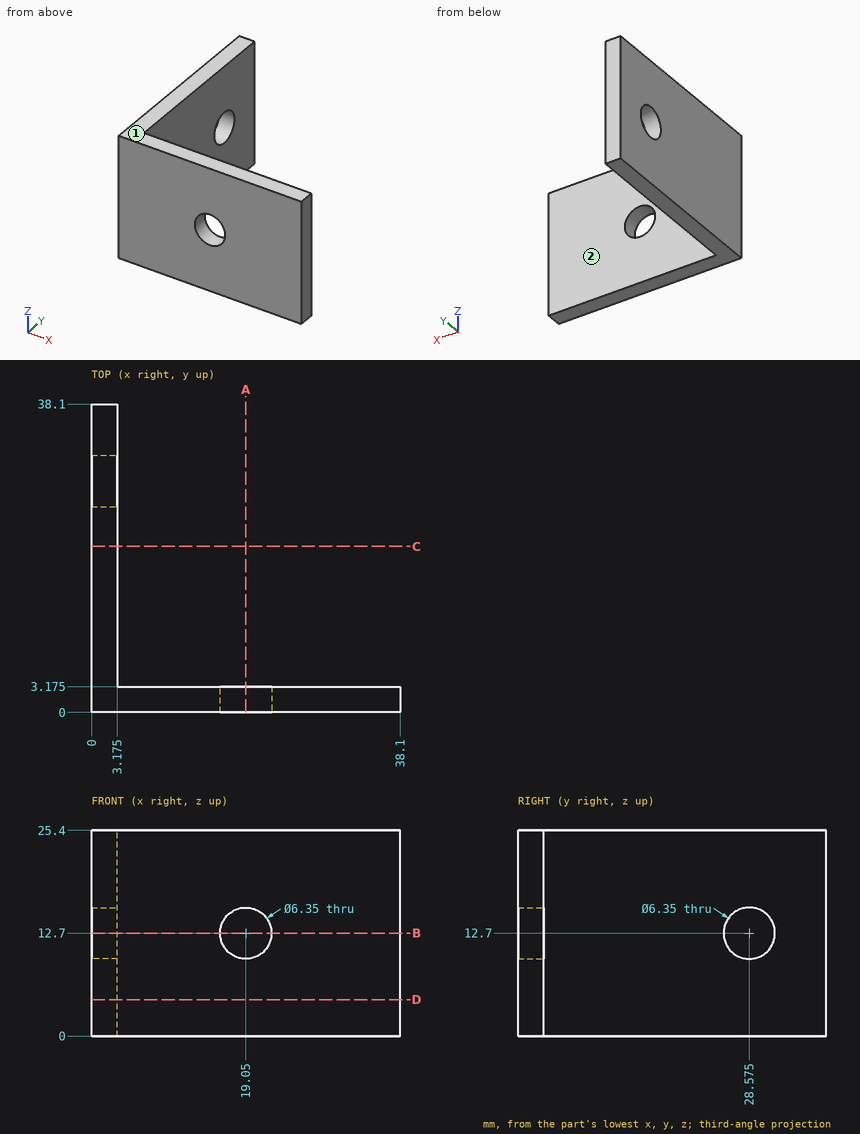
The drawing under review shows one solid part. Ordinate dimensions are in mm from its lowest x, y, z. A direction names the side the tool comes from. Coordinates: 2 decimals unless noted, no trailing zeros. Write each loop counter-clockwise with the first axis right and the second up, starting at its lowest first coordinate (ties: lowest second). Pieces come first, ordered by that corner, then holes. Notation, with made-up numbers: (44.5, 64) - (103.5, 64) arc R18 ccw to (103.5, 81) - close; hole circle Ø2 at (61.25, 84.5). An arc over 180 degrees is marked (long way). Answer as CSV lines item,"result".
(1) We need section C-C (y = 20.5). Give the boundary of the cut face in (x, z) (3 decimals).
Data:
outline,"(0, 0) - (3.175, 0) - (3.175, 25.4) - (0, 25.4) - close"
(2) Clearance check with flat-ended pins moving along their axes: pin 1 Ø12.5 at (x, z) = (21, 16.5) entering from +Y (3 decimals); pin 2 Ø5.5 at (x, z) = (19.05, 12.7) entering from +Y; pin 3 Ø7.5 at (y, z) = (28.575, 12.7) entering from +X (3 decimals); pin 4 Ø4 at (y, z) = (9, 9.5) entering from -X. State where each tip first meets the part, or that it passes through.
Data:
pin 1,"stops at y = 3.175"
pin 2,"passes through"
pin 3,"stops at x = 3.175"
pin 4,"stops at x = 0"
(3) Tool access review of the marked faces 1 and 2: name each direction out of +Z, -Z, +X, -X, +Y, -Y from which nothing blocks a thin tool from reaching the whole face with its end or side.
Data:
face 1,"+Z, +X, -X, +Y, -Y"
face 2,"+Z, -Z, +X, +Y"
(4) We need section D-D (z = 4.5). Give the boundary of the cut face in (x, y) (3 decimals).
Data:
outline,"(0, 0) - (38.1, 0) - (38.1, 3.175) - (3.175, 3.175) - (3.175, 38.1) - (0, 38.1) - close"
(5) We need section B-B (z = 12.7). Give the boundary of the cut face in (x, y) (3 decimals), plus the area to 3 significant figures.
Data:
outline,"(0, 0) - (15.875, 0) - (15.875, 3.175) - (3.175, 3.175) - (3.175, 25.4) - (0, 25.4) - close; (0, 31.75) - (3.175, 31.75) - (3.175, 38.1) - (0, 38.1) - close; (22.225, 0) - (38.1, 0) - (38.1, 3.175) - (22.225, 3.175) - close"
area,"192 mm2"
(6) For line 1 along Z through (x, y) = (19.05, 2.55) (3 decimals); line 2 along X through (y, z) = (34, 17) (3 decimals); line 3 along Y through (x, z) = (0.75, 12.7), list the stretches that pass through material, from the lowest coordinate up. Write a range as [from, to].
Data:
line 1,"z = [0, 9.525], [15.875, 25.4]"
line 2,"x = [0, 3.175]"
line 3,"y = [0, 25.4], [31.75, 38.1]"
(7) We need section A-A (x = 19.05). Give the boundary of the cut face in (y, z) (3 decimals).
Data:
outline,"(0, 0) - (3.175, 0) - (3.175, 9.525) - (0, 9.525) - close; (0, 15.875) - (3.175, 15.875) - (3.175, 25.4) - (0, 25.4) - close"
